Verification items for the finished model (mm, model axes). A direction names the side the tool comes from. Coordinates: 2 decimals unless noted, no trailing zeros. Write each loop counter-clockwise with the first axis right and the second up, starting at its lowest first coordinate (ties: lowest second). Pieces come first, ordered by that corner, then holes. Notation, with made-up numbers: (-31, 73.5) -> (18, 73.5) arc R23 cw to (18, 97.5) -> close; hole circle Ø1 at (2, 14.5). An arc over 180 degrees is marked (long way). Write item = value, one per line. Start each with the question number.
(1) Set-up check for faces 4 (the face through (-6, 80, 1)), 5 (the face through (-24, 82, 0)), 6 (the face through (-10, 140, 1)): record each of +Z, -Z, +X, -X, +Y, -Y from which the full face is reachable in a straight line by a thin tool's end or side.
(2) Section check C-C (y = 41). Record the cut outline in (x, z).
(3) Mould release check, pull along X, two halves, no side actions. Record for faces 1 (the face through (-21, 32, 1)), 2 (the face through (-20, 127, 1)), 3 (the face through (3, 150, 1)): released by +X, released by -X, zero draft, split by the parting line, or undercut.
(4) Section check D-D (z = 2.45). State how many separate pieces and enclosed holes the cut face has, plus the area to 3 significant figures.
(5) Material ranges on probe 1 along Y at (x, z) = (-6, 0.9); probe 2 along Y at (x, z) = (1.5, 0.7); probe 3 along Y at (x, z) = (-8.5, 0.65), recorded low to high. Write a range as [from, to].
(6) Gauge pin test, flat ends, axial feed: pin 1 Ø0.9 at (y, z) = (30.5, 1.5) entering from +X; pin 2 Ø4 at (x, y) = (1.5, 154) entering from +Z; pin 3 Ø1 at (y, z) = (18, 0.5) entering from +X. Record the tip position at first contact, or that the pin passes through.
(7) Section check A-A (x = 1.5). Record the cut outline in (y, z).
(8) Section check B-B (x = -24.5). Record the cut outline in (y, z), plus the area to 3 significant figures.
```python
from build123d import *

# Parameters (mm, degrees)
SKETCH_1_W      = 8
SKETCH_1_H      = 3
EXTRUDE_1_DEPTH = 3


with BuildPart() as part:
    # 草图1 → 凸台-拉伸1 (new body)
    with BuildSketch(Plane.XY):
        with BuildLine():
            Line((0, 140), (0, 146))
            Line((0, 146), (3, 146))
            Line((3, 146), (3, 153.609487516))
            ThreePointArc((3, 153.609487516), (-0.05, 154), (3, 154.390512484))
            Line((3, 154.390512484), (3, 162))
            Line((3, 162), (0, 162))
            Line((0, 162), (-51, 162))
            Line((-51, 162), (-51, 0))
            Line((-51, 0), (0, 0))
            Line((0, 0), (3, 0))
            Line((3, 0), (3, 7.609487516))
            ThreePointArc((3, 7.609487516), (-0.05, 8), (3, 8.390512484))
            Line((3, 8.390512484), (3, 16))
            Line((3, 16), (0, 16))
            Line((0, 16), (-15, 16))
            Line((-15, 16), (-15, 29))
            Line((-15, 29), (-18, 29))
            Line((-18, 29), (-26, 29))
            Line((-26, 29), (-26, 32))
            Line((-26, 32), (-18, 32))
            Line((-18, 32), (-15, 32))
            Line((-15, 32), (-15, 45))
            Line((-15, 45), (0, 45))
            Line((0, 45), (3, 45))
            Line((3, 45), (3, 76))
            Line((3, 76), (0, 76))
            Line((0, 76), (0, 82))
            Line((0, 82), (-5, 82))
            Line((-5, 82), (-5, 80))
            Line((-5, 80), (-8, 80))
            Line((-8, 80), (-8, 82))
            Line((-8, 82), (-12, 82))
            Line((-12, 82), (-12, 86))
            Line((-12, 86), (-8, 86))
            Line((-8, 86), (-8, 88))
            Line((-8, 88), (-5, 88))
            Line((-5, 88), (-5, 86))
            Line((-5, 86), (0, 86))
            Line((0, 86), (0, 92))
            Line((0, 92), (3, 92))
            Line((3, 92), (3, 130))
            Line((3, 130), (0, 130))
            Line((0, 130), (0, 136))
            Line((0, 136), (-5, 136))
            Line((-5, 136), (-5, 134))
            Line((-5, 134), (-8, 134))
            Line((-8, 134), (-8, 136))
            Line((-8, 136), (-12, 136))
            Line((-12, 136), (-12, 140))
            Line((-12, 140), (-8, 140))
            Line((-8, 140), (-8, 142))
            Line((-8, 142), (-5, 142))
            Line((-5, 142), (-5, 140))
            Line((-5, 140), (0, 140))
        make_face()
        with Locations((-22, 54.5)):
            Rectangle(SKETCH_1_W, SKETCH_1_H, mode=Mode.SUBTRACT)
        Polygon((-11, 125), (-8, 125), (-8, 130), (-5, 130), (-5, 120), (-32, 120), (-32, 130), (-29, 130), (-29, 125), (-26, 125), (-26, 130), (-23, 130), (-23, 125), (-20, 125), (-20, 130), (-17, 130), (-17, 125), (-14, 125), (-14, 130), (-11, 130), align=None, mode=Mode.SUBTRACT)
    extrude(amount=EXTRUDE_1_DEPTH)


solid = part.part
```
Response:
q1.face_4 = +Z, -Z
q1.face_5 = -Z, +X, -X, +Y, -Y
q1.face_6 = +Z, -Z, +X
q2.outline = (-51, 0) -> (-15, 0) -> (-15, 3) -> (-51, 3) -> close
q3.face_1 = zero draft
q3.face_2 = undercut
q3.face_3 = released by +X
q4.separate_pieces = 1
q4.enclosed_holes = 2
q4.area = 7,730 mm2
q5.probe_1 = [0, 16], [45, 80], [88, 120], [130, 134], [142, 162]
q5.probe_2 = [0, 6.45], [9.55, 16], [45, 76], [92, 130], [146, 152.45], [155.55, 162]
q5.probe_3 = [0, 16], [45, 82], [86, 120], [125, 136], [140, 162]
q6.pin_1 = -26
q6.pin_2 = 3
q6.pin_3 = -15
q7.outline = (0, 0) -> (6.45, 0) -> (6.45, 3) -> (0, 3) -> close; (9.55, 0) -> (16, 0) -> (16, 3) -> (9.55, 3) -> close; (45, 0) -> (76, 0) -> (76, 3) -> (45, 3) -> close; (92, 0) -> (130, 0) -> (130, 3) -> (92, 3) -> close; (146, 0) -> (152.45, 0) -> (152.45, 3) -> (146, 3) -> close; (155.55, 0) -> (162, 0) -> (162, 3) -> (155.55, 3) -> close
q8.outline = (0, 0) -> (29, 0) -> (29, 3) -> (0, 3) -> close; (32, 0) -> (53, 0) -> (53, 3) -> (32, 3) -> close; (56, 0) -> (120, 0) -> (120, 3) -> (56, 3) -> close; (130, 0) -> (162, 0) -> (162, 3) -> (130, 3) -> close
q8.area = 438 mm2
